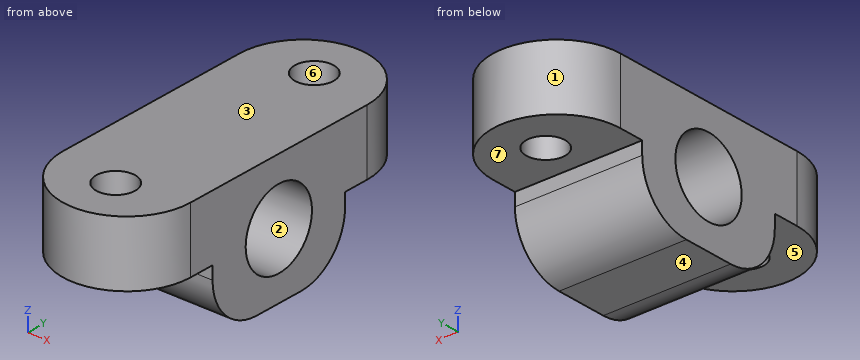
from build123d import *

# Parameters (mm, degrees)
PAD_DEPTH       = 5
SKETCH001_W     = 9.862508
SKETCH001_H     = 12
PAD001_DEPTH    = 10
SKETCH002_R     = 3
POCKET_DEPTH    = 9.863573
SKETCH003_R     = 1.5
POCKET001_DEPTH = 5
FILLET_R        = 4


with BuildPart() as part:
    # Sketch → Pad (new body)
    with BuildSketch(Plane.XY):
        with BuildLine():
            Line((138.65243, 91.791451), (138.65243, 75.79029))
            ThreePointArc((138.65243, 75.79029), (143.608931, 70.884283), (148.514938, 75.840785))
            Line((148.514938, 91.791451), (148.514938, 75.840785))
            ThreePointArc((148.514938, 91.791451), (143.583684, 96.722705), (138.65243, 91.791451))
        make_face()
    extrude(amount=PAD_DEPTH)

    # Sketch001 → Pad001 (join)
    with BuildSketch(Plane.XY.offset(5)):
        with Locations((143.583684, 83.816118)):
            Rectangle(SKETCH001_W, SKETCH001_H)
    extrude(amount=-PAD001_DEPTH)

    # Sketch002 (on Face9 of Pad001) → Pocket (cut, through all)
    with BuildSketch(Plane(origin=(138.65243, 0, 0), x_dir=(0, -1, 0), z_dir=(-1, 0, 0))):
        with Locations((-83.816118, 0)):
            Circle(SKETCH002_R)
    extrude(amount=-POCKET_DEPTH, mode=Mode.SUBTRACT)

    # Sketch003 (on Face10 of Pocket) → Pocket001 (cut)
    with BuildSketch(Plane(origin=(0, 0, 0), x_dir=(1, 0, 0), z_dir=(0, 0, -1))):
        with Locations((143.583684, -74.815537)):
            Circle(SKETCH003_R)
        with Locations((143.583684, -92.791451)):
            Circle(SKETCH003_R)
    extrude(amount=-POCKET001_DEPTH, mode=Mode.SUBTRACT)

    # Fillet
    fillet_edges = [part.edges().sort_by_distance(p)[0] for p in [
        (143.583684, 89.816118, -5),
        (143.583684, 77.816118, -5),
    ]]
    fillet(fillet_edges, radius=FILLET_R)


solid = part.part
For this review, take the finished solid that the model builds, in its own axes (mm). Face numbers are marked on the shaded views. A direction names the side the tool comes from. Round coordinates to 2 decimals unless told otherwise and drop trailing zeros. Write each loop counter-clockwise with the first axis right and the second up, starting at its lowest first coordinate (ties: lowest second). Pieces come first, ordered by that corner, then holes. Notation, with made-up numbers: M 31.5,72.5 L 48.5,72.5 A22 ccw 48.5,104.5 Z; hole C -39.75,-37 d2. An arc over 180 degrees is marked long. Write item = value, one per line. Start each with the question number.
(1) We need section C-C (y = 75.5). Give the boundary of the cut face in (x, z), then the cut area to 3 significant figures.
(2) For the marked faces 5, 6 and 7, list the 3-axis set-ups (+Z, -Z, +X, -X, +Y, -Y) from which the entire face can be reached by the end or side of a thin tool; tool diameter is ignored.
(3) We need section A-A (z = 1.5). Give the boundary of the cut face in (x, y).
(4) Clearance check with flat-ended pins moving along their axes: pin 1 Ø1.5 at (x, y) = (145, 76.5) entering from -Z; pin 2 Ø1 at (x, z) = (144.5, -3) entering from -Y; pin 3 Ø0.5 at (x, z) = (141.5, -0.5) entering from +Y. State where each tip first meets the part, or that it passes through.
(5) For line 1 along Z through (x, y) = (143, 76.25); line 2 along Y through (x, z) = (143.25, 4.5); line 3 along X through (y, z) = (91.75, 1), list the stretches that pass through material, from the lowest coordinate up.
(6) We need section D-D (z = -0.75). Give the boundary of the cut face in (x, y).
(7) We need section B-B (x = 144.5). Give the boundary of the cut face in (y, z).
(8) The part is to be moulded in two halves that separate along Z. For the marked faces 1, 2, 3 and 4, say which applies: +Z half, -Z half, draft (parallel to the pull), parting line (faces both ways), or undercut.
Results found:
q1.outline = M 138.66,0 L 142.25,0 L 142.25,5 L 138.66,5 Z; M 144.92,0 L 148.5,0 L 148.5,5 L 144.92,5 Z
q1.area = 35.9 mm²
q2.face_5 = -Z, +X, -X, -Y
q2.face_6 = +Z, -Z
q2.face_7 = -Z, +X, -X, +Y
q3.outline = M 138.65,75.79 A4.93 ccw 148.51,75.84 L 148.51,81.22 L 138.65,81.22 Z; M 138.65,86.41 L 148.51,86.41 L 148.51,91.79 A4.93 ccw 138.65,91.79 Z; hole C 143.58,74.82 d3; hole C 143.58,92.79 d3
q4.pin_1 = 0
q4.pin_2 = 78.11
q4.pin_3 = 89.82
q5.line_1 = 0 to 5
q5.line_2 = 70.9 to 73.35, 76.28 to 91.33, 94.25 to 96.71
q5.line_3 = 138.65 to 142.5, 144.66 to 148.51
q6.outline = M 138.65,77.82 L 148.51,77.82 L 148.51,80.91 L 138.65,80.91 Z; M 138.65,86.72 L 148.51,86.72 L 148.51,89.82 L 138.65,89.82 Z
q7.outline = M 70.97,0 L 73.63,0 L 73.63,5 L 70.97,5 Z; M 76,0 L 77.82,0 L 77.82,-1 A4 ccw 81.82,-5 L 85.82,-5 A4 ccw 89.82,-1 L 89.82,0 L 91.6,0 L 91.6,5 L 76,5 Z; M 93.98,0 L 96.64,0 L 96.64,5 L 93.98,5 Z; hole C 83.82,0 d6
q8.face_1 = draft
q8.face_2 = undercut
q8.face_3 = +Z half
q8.face_4 = -Z half
